The listing builds one solid part. Answer for the finished solid, in the listing's coordinates (mm). A direction names the side the tool comes from. Round coordinates to 2 decimals unless told otherwise and drop trailing zeros. Loops run counter-clockwise (first coordinate to the right, second up) from the corner with the lowest first, then second, coordinate; pieces in that order, holes last. Notation, with made-up numbers: (-15.5, 42) - (2.5, 42) arc R33 cw to (2.5, 77) - close; hole circle Ø1 at (-21, 37). An arc over 180 degrees is marked (long way). Write item = value, one per line. Start each with the question number.
1) Section A-A, the plane y = -0.25 is taken. Determine the outline of the cut face in (x, z).
2) Section C-C, the plane z = 1 is taken. Determine the outline of the cut face in (x, y), and give its area (3 significant figures).
3) A tool of negligible diameter and unlimited length cuts with its end or side. For faces 4 (the cylindrical face through (4.8, -1, -4.8)), 5 (the cylindrical face through (-2.8, 3.3, 0.1)), 6 (the flat face through (2, -1.8, 3)), from which of +Z, -Z, +X, -X, +Y, -Y can it reach the whole face along a straight path? Write none if from no direction.
4) Section D-D, the plane x = 4.75 is taken. Determine the outline of the cut face in (y, z).
5) For a pull along Z with two mould halves and no side action, classify faces 1 (the flat face through (5, -1.8, 1)), 2 (the flat face through (0, -1, -6)), 3 (the flat face through (0, 6.5, 0)) as released by +Z, released by -Z, zero draft, split by the parting line, or undercut.
6) Section B-B, the plane x = 1.75 is taken. Determine the outline of the cut face in (y, z), and give its area (3 significant figures).
7) Straight lines are drawn through the part: line 1 along X through (y, z) = (5.5, 0); line 2 along Y through (x, z) = (-3, 3.5); line 3 along Y through (x, z) = (0.5, -2.5). For each, find the intervals that lie inside material, in ascending order.
8) Given pin 1 Ø2 at (x, y) = (1.5, -0.5) entering from +Z; pin 2 Ø2.5 at (x, z) = (-2, 3.5) entering from -Y; pin 3 Ø1 at (x, z) = (3, -3.5) entering from +Y; pin 4 Ø2 at (y, z) = (2, 0) entering from +X, each flat-ended and moving along its own axis, determine where each tip first touches the part or whether it passes through.
from build123d import *

# Parameters (mm, degrees)
CYLINDER004_R     = 2.8
CYLINDER004_DEPTH = 7.5
PAD010_DEPTH      = 2
SKETCH037_R       = 1.5
POCKET008_DEPTH   = 0.2


with BuildPart() as part:
    # Cylinder004 → Cylinder004 (join)
    with BuildSketch(Plane.XZ.offset(-6.5)):
        Circle(CYLINDER004_R)
    extrude(amount=CYLINDER004_DEPTH)

    # Sketch036 → Pad010 (join)
    with BuildSketch(Plane.XZ):
        with BuildLine():
            ThreePointArc((-4.359163, 3.126626), (-6.630007, 0.874403), (-5.228622, -2.000551))
            ThreePointArc((-5.228622, -2.000551), (-4.849321, -4.732289), (-2.4, -6))
            Line((-2.4, -6), (2.4, -6))
            ThreePointArc((2.4, -6), (4.849321, -4.732289), (5.228622, -2.000551))
            ThreePointArc((5.228622, -2.000551), (6.630007, 0.874403), (4.359163, 3.126626))
            ThreePointArc((4.359163, 3.126626), (2.731228, 5.340757), (0, 5.035887))
            ThreePointArc((0, 5.035887), (-2.731228, 5.340757), (-4.359163, 3.126626))
        make_face()
    extrude(amount=PAD010_DEPTH)

    # Sketch037 → Pocket008 (cut)
    with BuildSketch(Plane(origin=(0, -2, -1), x_dir=(1, 0, 0), z_dir=(0, -1, 0))):
        with Locations((-4.565071, 1.483282)):
            Circle(SKETCH037_R)
        with Locations((4.565071, 1.483282)):
            Circle(SKETCH037_R)
        with Locations((-1.952336, 4.385018)):
            Circle(SKETCH037_R)
        with Locations((1.952336, 4.385018)):
            Circle(SKETCH037_R)
        with BuildLine():
            ThreePointArc((2.594039, 1.054023), (0, 2.8), (-2.594039, 1.054023))
            ThreePointArc((-3.699936, -0.480077), (-3.055021, 0.220676), (-2.594039, 1.054023))
            ThreePointArc((-3.699936, -0.480077), (-4.22241, -2.823905), (-2.117647, -3.979969))
            ThreePointArc((2.117647, -3.979969), (0, -3.829736), (-2.117647, -3.979969))
            ThreePointArc((2.117647, -3.979969), (4.22241, -2.823905), (3.699936, -0.480077))
            ThreePointArc((2.594039, 1.054023), (3.055021, 0.220676), (3.699936, -0.480077))
        make_face()
    extrude(amount=-POCKET008_DEPTH, mode=Mode.SUBTRACT)


solid = part.part
Geometry check:
q1.outline = (-5.23, -2) arc R3 ccw to (-2.4, -6) - (2.4, -6) arc R3 ccw to (5.23, -2) arc R2.75 ccw to (4.36, 3.13) arc R2.75 ccw to (0, 5.04) arc R2.75 ccw to (-4.36, 3.13) arc R2.75 ccw to start
q2.outline = (-6.61, -2) - (-5.97, -2) - (-5.97, -1.8) - (-3.16, -1.8) - (-3.16, -2) - (-1.96, -2) - (-1.96, -1.8) - (1.96, -1.8) - (1.96, -2) - (3.16, -2) - (3.16, -1.8) - (5.97, -1.8) - (5.97, -2) - (6.61, -2) - (6.61, 0) - (2.62, 0) - (2.62, 6.5) - (-2.62, 6.5) - (-2.62, 0) - (-6.61, 0) - close
q2.area = 58.5 mm2
q3.face_4 = +X, +Y, -Y
q3.face_5 = +Y
q3.face_6 = -Y
q4.outline = (-2, -4.86) - (0, -4.86) - (0, 3.03) - (-2, 3.03) - (-2, 1.97) - (-1.8, 1.97) - (-1.8, -1.01) - (-2, -1.01) - close
q5.face_1 = undercut
q5.face_2 = released by -Z
q5.face_3 = zero draft
q6.outline = (-2, -6) - (0, -6) - (0, -2.19) - (6.5, -2.19) - (6.5, 2.19) - (0, 2.19) - (0, 5.57) - (-2, 5.57) - (-2, 4.87) - (-1.8, 4.87) - (-1.8, 1.9) - (-2, 1.9) - (-2, 1.19) - (-1.8, 1.19) - (-1.8, -4.93) - (-2, -4.93) - close
q6.area = 49.7 mm2
q7.line_1 = -2.8 to 2.8
q7.line_2 = -1.8 to 0
q7.line_3 = -1.8 to 6.5
q8.pin_1 = 5.57
q8.pin_2 = -1.8
q8.pin_3 = 0
q8.pin_4 = 2.8
